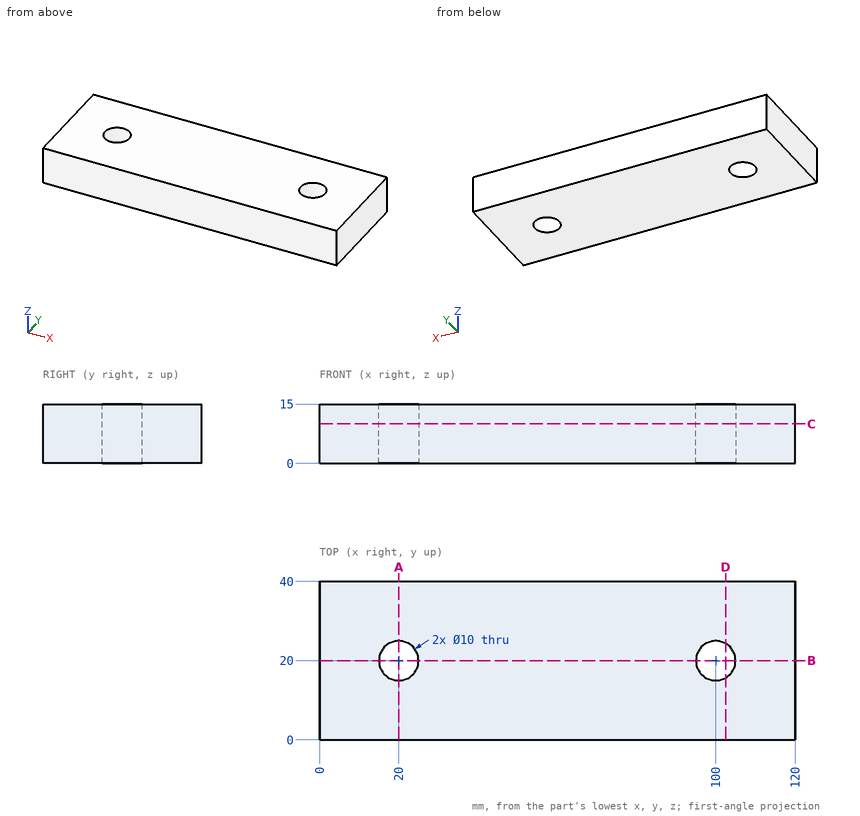
Check sheet for the drawn part. Datum: minimum x, y, z corner. Units: mm. Coordinates: 2 decimals unless noted, no trailing zeros. Loops run counter-clockwise (first coordinate to the right, second up) from the corner with the lowest first, then second, coordinate; pieces in that order, holes last. Notation, with made-up numbers: (58.25, -23) -> (71.25, -23) arc R23 ccw to (71.25, -3) -> close; hole circle Ø3 at (54, 2). An arc over 180 degrees is marked (long way). Answer in a Markdown table with one row per item.
1) Scan lines: line 1 along Y through (x, z) = (100, 4.25); line 2 along X through (y, z) = (19, 6.5); line 3 along X through (y, z) = (18, 3.5). Record each from-to range of solid material in increasing order. Write a range as from..to.
The answers:
| item | result |
|---|---|
| line 1 | y = 0..15, 25..40 |
| line 2 | x = 0..15.1, 24.9..95.1, 104.9..120 |
| line 3 | x = 0..15.42, 24.58..95.42, 104.58..120 |
2) Section check B-B (y = 20). Record the cut outline in (x, z).
The answers:
| item | result |
|---|---|
| outline | (0, 0) -> (15, 0) -> (15, 15) -> (0, 15) -> close; (25, 0) -> (95, 0) -> (95, 15) -> (25, 15) -> close; (105, 0) -> (120, 0) -> (120, 15) -> (105, 15) -> close |
3) Section check A-A (x = 20). Record the cut outline in (y, z), and give its area (3 significant figures).
The answers:
| item | result |
|---|---|
| outline | (0, 0) -> (15, 0) -> (15, 15) -> (0, 15) -> close; (25, 0) -> (40, 0) -> (40, 15) -> (25, 15) -> close |
| area | 450 mm2 |
4) Section check C-C (z = 10). Record the cut outline in (x, y), and give its area (3 significant figures).
The answers:
| item | result |
|---|---|
| outline | (0, 0) -> (120, 0) -> (120, 40) -> (0, 40) -> close; hole circle Ø10 at (20, 20); hole circle Ø10 at (100, 20) |
| area | 4,640 mm2 |
5) Section check D-D (x = 102.5). Record the cut outline in (y, z), and give its area (3 significant figures).
The answers:
| item | result |
|---|---|
| outline | (0, 0) -> (15.67, 0) -> (15.67, 15) -> (0, 15) -> close; (24.33, 0) -> (40, 0) -> (40, 15) -> (24.33, 15) -> close |
| area | 470 mm2 |
